from build123d import *

# Parameters (mm, degrees)
EXTRUDE_1_DEPTH     = 3
SKETCH_3_R          = 1.5
CUT_EXTRUDE_2_DEPTH = 3
SKETCH_4_R          = 2
CUT_EXTRUDE_3_DEPTH = 3


with BuildPart() as part:
    # 草图2 → 凸台-拉伸1 (new body)
    with BuildSketch(Plane.XY):
        Polygon((-85, 40), (-80, 40), (-80, 43), (-70, 43), (-70, 40), (-65, 40), (-65, 43), (-55, 43), (-55, 40), (-50, 40), (-50, 43), (-40, 43), (-40, 40), (-35, 40), (-35, 43), (-25, 43), (-25, 40), (-20, 40), (-20, 43), (-10, 43), (-10, 40), (-5, 40), (-5, 43), (5, 43), (5, 40), (10, 40), (10, 43), (20, 43), (20, 40), (25, 40), (25, 43), (35, 43), (35, 40), (40, 40), (40, 43), (50, 43), (50, 40), (55, 40), (55, 43), (65, 43), (65, 40), (70, 40), (70, 43), (80, 43), (80, 40), (85, 40), (85, 35), (88, 35), (88, 25), (85, 25), (85, 20), (88, 20), (88, 10), (85, 10), (85, 5), (88, 5), (88, -5), (85, -5), (85, -10), (88, -10), (88, -20), (85, -20), (85, -25), (88, -25), (88, -35), (85, -35), (85, -40), (80, -40), (80, -43), (70, -43), (70, -40), (65, -40), (65, -43), (55, -43), (55, -40), (50, -40), (50, -43), (40, -43), (40, -40), (35, -40), (35, -43), (25, -43), (25, -40), (20, -40), (20, -43), (10, -43), (10, -40), (5, -40), (5, -43), (-5, -43), (-5, -40), (-10, -40), (-10, -43), (-20, -43), (-20, -40), (-25, -40), (-25, -43), (-35, -43), (-35, -40), (-40, -40), (-40, -43), (-50, -43), (-50, -40), (-55, -40), (-55, -43), (-65, -43), (-65, -40), (-70, -40), (-70, -43), (-80, -43), (-80, -40), (-85, -40), (-85, -35), (-88, -35), (-88, -25), (-85, -25), (-85, -20), (-88, -20), (-88, -10), (-85, -10), (-85, -5), (-88, -5), (-88, 5), (-85, 5), (-85, 10), (-88, 10), (-88, 20), (-85, 20), (-85, 25), (-88, 25), (-88, 35), (-85, 35), align=None)
    extrude(amount=EXTRUDE_1_DEPTH)

    # 草图3 → 切除-拉伸2 (cut)
    with BuildSketch(Plane.XY.offset(3)):
        with Locations((-32.5, 16.5)):
            Circle(SKETCH_3_R)
        with Locations((32.5, 16.5)):
            Circle(SKETCH_3_R)
        with Locations((32.5, -16.5)):
            Circle(SKETCH_3_R)
        with Locations((-32.5, -16.5)):
            Circle(SKETCH_3_R)
    extrude(amount=-CUT_EXTRUDE_2_DEPTH, mode=Mode.SUBTRACT)

    # 草图4 → 切除-拉伸3 (cut)
    with BuildSketch(Plane.XY.offset(3)):
        with Locations((78, 0)):
            Circle(SKETCH_4_R)
        with Locations((-78, 0)):
            Circle(SKETCH_4_R)
    extrude(amount=-CUT_EXTRUDE_3_DEPTH, mode=Mode.SUBTRACT)


solid = part.part
The listing builds one solid part. Answer for the finished solid, in the listing's coordinates (mm). A direction names the side the tool comes from. Coordinates: 2 decimals unless noted, no trailing zeros. Order: outer loops, then holes, each group sorted by start corner. A loop starts at its lowest first (then second) coordinate and runs counter-clockwise, first axis right, second up. Notation, with made-up numbers: (37.5, 50.25) -> (92.5, 50.25) arc R25 ccw to (92.5, 70.25) -> close; hole circle Ø11 at (-37, 46). An arc over 180 degrees is marked (long way). Answer in a Markdown table with one row per item. Add a question column.
Item 1: Find the intervals of material crossed by L1, parallel to Y at x = -32.5, z = 1.8; L2, parallel to Y at x = 31.5, z = 2.35; L3, parallel to Y at x = -78, z = 1.4, in increasing order. Write a range as from..to.
Item 2: Determine the mould class of faces 5 (the face through (40, 41, 1)), 6 (the face through (-37, -40, 1)), 7 (the face through (85, 8, 1)) for opening direction Y: +Y half, -Y half, draft (parallel to the pull), parting line (faces both ways), or undercut.
Item 3: Which of the six approach directions +Z, -Z, +X, -X, +Y, -Y give full straight-line access (tool end or side, diameter ignored) to faces 1 (the face through (86, -10, 1)), 2 (the face through (5, -41, 1)), 3 (the face through (86, 35, 1)), 4 (the face through (-8, 40, 1))?
Item 4: Each of these flat-tipped pins is pushed along its axis until it touches: P1, Ø0.9, axis at y = 7.5, z = 1, coming from the -X side; P2, Ø1.5, axis at x = -86.5, z = 1, coming from the -Y side; P3, Ø1.5, axis at x = 7, z = 1, coming from the +Y side. Where does it stop, or does it pass through?
Item 5: Find section C-C (z = 0.6). State how many separate pieces and enclosed holes the cut face has, then the cut area to 3 significant figures.
Item 6: Find section B-B (x = -78). Write down the section's boundary in (y, z), then the cut area to 3 significant figures.
Item 7: Find section A-A (y = 0). Write down the section's boundary in (x, z), then the cut area to 3 significant figures.
Result set:
| question | item | result |
|---|---|---|
| 1 | L1 | y = -43..-18, -15..15, 18..43 |
| 1 | L2 | y = -43..-17.62, -15.38..15.38, 17.62..43 |
| 1 | L3 | y = -43..-2, 2..43 |
| 2 | face 5 | draft |
| 2 | face 6 | -Y half |
| 2 | face 7 | undercut |
| 3 | face 1 | +Z, -Z, +X |
| 3 | face 2 | +Z, -Z, -Y |
| 3 | face 3 | +Z, -Z, +X, +Y |
| 3 | face 4 | +Z, -Z, +Y |
| 4 | P1 | stops at x = -85 |
| 4 | P2 | stops at y = -35 |
| 4 | P3 | stops at y = 40 |
| 5 | separate pieces | 1 |
| 5 | enclosed holes | 6 |
| 5 | area | 14,500 mm² |
| 6 | outline | (-43, 0) -> (-2, 0) -> (-2, 3) -> (-43, 3) -> close; (2, 0) -> (43, 0) -> (43, 3) -> (2, 3) -> close |
| 6 | area | 246 mm² |
| 7 | outline | (-88, 0) -> (-80, 0) -> (-80, 3) -> (-88, 3) -> close; (-76, 0) -> (76, 0) -> (76, 3) -> (-76, 3) -> close; (80, 0) -> (88, 0) -> (88, 3) -> (80, 3) -> close |
| 7 | area | 504 mm² |
